from build123d import *

# Parameters (mm, degrees)
SKETCH_1_R          = 24
EXTRUDE_1_DEPTH     = 7
SKETCH_2_R          = 17
EXTRUDE_2_DEPTH     = 23
CUT_EXTRUDE_1_DEPTH = 23
CUT_EXTRUDE_3_REACH = 47.299
SKETCH_4_W          = 24
SKETCH_4_H          = 8.031532799
SKETCH_5_R          = 2
CUT_EXTRUDE_2_DEPTH = 42


with BuildPart() as part:
    # Эскиз1 → Вытянуть1 (new body)
    with BuildSketch(Plane(origin=(0, 0, 0), x_dir=(1, 0, 0), z_dir=(0, 1, 0))):
        with Locations(Location((0, 0, 0), (0, 0, 270))):
            Circle(SKETCH_1_R)
    extrude(amount=EXTRUDE_1_DEPTH)

    # Эскиз2 → Вытянуть2 (add)
    with BuildSketch(Plane(origin=(0, 7, 0), x_dir=(1, 0, 0), z_dir=(0, 1, 0))):
        with Locations(Location((0, 0, 0), (0, 0, 270))):
            Circle(SKETCH_2_R)
    extrude(amount=EXTRUDE_2_DEPTH)

    # Эскиз3 → Вырез-Вытянуть1 (cut, symmetric)
    with BuildSketch(Plane.XY):
        with BuildLine():
            Line((-7, 24.269678179), (7, 24.269678179))
            ThreePointArc((7, 24.269678179), (12, 19.269678179), (7, 14.269678179))
            Line((7, 14.269678179), (-7, 14.269678179))
            ThreePointArc((-7, 14.269678179), (-12, 19.269678179), (-7, 24.269678179))
        make_face()
    extrude(amount=CUT_EXTRUDE_1_DEPTH, both=True, mode=Mode.SUBTRACT)

    # Вытянуть3: up to this face of the body (flat: up to its plane)
    cut_extrude_3_end = Plane(part.part.faces().sort_by_distance((0, 7, -23.32117749))[0])
    # Эскиз4 → Вытянуть3 (cut, up to the picked face)
    with BuildSketch(Plane(origin=(0, 30, 0), x_dir=(-1, 0, 0), z_dir=(0, 1, 0)), mode=Mode.PRIVATE) as cut_extrude_3_sk1:
        with Locations((0, -16.0157664)):
            Rectangle(SKETCH_4_W, SKETCH_4_H)
    cut_extrude_3_tool1 = split(extrude(cut_extrude_3_sk1.sketch, amount=-CUT_EXTRUDE_3_REACH, mode=Mode.PRIVATE), bisect_by=cut_extrude_3_end, keep=Keep.BOTH, mode=Mode.PRIVATE)
    # Эскиз4 → Вытянуть3 (cut, up to the picked face)
    with BuildSketch(Plane(origin=(0, 30, 0), x_dir=(-1, 0, 0), z_dir=(0, 1, 0)), mode=Mode.PRIVATE) as cut_extrude_3_sk2:
        with Locations((0, 16.0157664)):
            Rectangle(SKETCH_4_W, SKETCH_4_H)
    cut_extrude_3_tool2 = split(extrude(cut_extrude_3_sk2.sketch, amount=-CUT_EXTRUDE_3_REACH, mode=Mode.PRIVATE), bisect_by=cut_extrude_3_end, keep=Keep.BOTH, mode=Mode.PRIVATE)
    add(cut_extrude_3_tool1.solids().sort_by(Axis((0, 30, -16.015766), (0, -1, 0)))[0], mode=Mode.SUBTRACT)
    add(cut_extrude_3_tool2.solids().sort_by(Axis((0, 30, 16.015766), (0, -1, 0)))[0], mode=Mode.SUBTRACT)

    # Эскиз5 → Вырез-Вытянуть2 (cut, through all)
    with BuildSketch(Plane(origin=(0, 7, 0), x_dir=(1, 0, 0), z_dir=(0, 1, 0))):
        with Locations(Location((0, 20, 0), (0, 0, 270))):
            Circle(SKETCH_5_R)
        with Locations(Location((17.320508076, 10, 0), (0, 0, 270))):
            Circle(SKETCH_5_R)
        with Locations(Location((17.320508076, -10, 0), (0, 0, 270))):
            Circle(SKETCH_5_R)
        with Locations(Location((0, -20, 0), (0, 0, 270))):
            Circle(SKETCH_5_R)
        with Locations(Location((-17.320508076, -10, 0), (0, 0, 270))):
            Circle(SKETCH_5_R)
        with Locations(Location((-17.320508076, 10, 0), (0, 0, 270))):
            Circle(SKETCH_5_R)
    extrude(amount=-CUT_EXTRUDE_2_DEPTH, mode=Mode.SUBTRACT)


solid = part.part
Can you work these out from the model? Positions are in its coordinate system, mm. A direction names the side the tool comes from. Round coordinates to 2 decimals unless told otherwise and drop trailing zeros. Loops run counter-clockwise (first coordinate to the right, second up) from the corner with the lowest first, then second, coordinate; pieces in that order, holes last. Notation, with made-up numbers: (-6, -32.75) - (12, -32.75) arc R23 ccw to (12, -9.75) - close; hole circle Ø4 at (89, 4). An arc over 180 degrees is marked (long way). Answer in a Markdown table with one row per item. Add a question column.
Q1. I want a section at C-C on x = 18.5. List the corners of the cut face in (y, z) for me, and give its area (3 significant figures).
Q2. For pin 1 Ø2 at (y, z) = (3, 3) entering from +X; pin 2 Ø5 at (x, z) = (0, 20) entering from +Y; pin 3 Ø3 at (x, y) = (1, 25) entering from +Z, each with a flat end and sliding along its axis, tell me the tip position at first contact or that it passes through.
Q3. I need wall thicknesses on L1, parallel to Y at x = 6.5, z = -2.5; L2, parallel to X at y = 6.5, z = 10.5; L3, parallel to Y at x = -6, z = 21.5. Which ranges of each line are inside material? Lowest first, please.
Q4. I want a section at D-D on z = 19. List the corners of the cut face in (x, y) for me, and give its area (3 significant figures).
Q5. Which directions (+Z, -Z, +X, -X, +Y, -Y) give clear straight access to the entire face, cutting with the end or side of a thin tool? Please do faces 4 (the flat face through (0, 24.27, 0)), 5 (the cylindrical face through (-17, 18, 0)).
Q6. We'd pull the mould along Y, two halves only. Please class faces 1 (the cylindrical face through (12, 19.4, 0.2)), 2 (the flat face through (0, 0, 0)), 3 (the cylindrical face through (17, 18, 0)): pulls with the +Y half, pulls with the -Y half, needs draft (parallel to the pull), parting line crosses it, or undercut.
Q7. I want a section at B-B on x = 0. List the corners of the cut face in (y, z) for me, and give its area (3 significant figures).
Q8. I want a section at A-A on z = -10. List the corners of the cut face in (x, y) for me, and give its area (3 significant figures).
A:
| question | item | result |
|---|---|---|
| 1 | outline | (0, -15.29) - (7, -15.29) - (7, -11.62) - (0, -11.62) - close; (0, -8.38) - (7, -8.38) - (7, 8.38) - (0, 8.38) - close; (0, 11.62) - (7, 11.62) - (7, 15.29) - (0, 15.29) - close |
| 1 | area | 169 mm^2 |
| 2 | pin 1 | x = 23.92 |
| 2 | pin 2 | y = 7 |
| 2 | pin 3 | z = 12 |
| 3 | L1 | 0 to 14.27, 24.27 to 30 |
| 3 | L2 | -21.58 to -19.26, -15.38 to 15.38, 19.26 to 21.58 |
| 3 | L3 | 0 to 7 |
| 4 | outline | (-14.66, 0) - (-1.73, 0) - (-1.73, 7) - (-14.66, 7) - close; (1.73, 0) - (14.66, 0) - (14.66, 7) - (1.73, 7) - close |
| 4 | area | 181 mm^2 |
| 5 | face 4 | +Z, -Z |
| 5 | face 5 | -X, +Y |
| 6 | face 1 | undercut |
| 6 | face 2 | pulls with the -Y half |
| 6 | face 3 | needs draft |
| 7 | outline | (0, -24) - (7, -24) - (7, -22) - (0, -22) - close; (0, -18) - (7, -18) - (7, -12) - (14.27, -12) - (14.27, 12) - (7, 12) - (7, 18) - (0, 18) - close; (0, 22) - (7, 22) - (7, 24) - (0, 24) - close; (24.27, -12) - (30, -12) - (30, 12) - (24.27, 12) - close |
| 7 | area | 592 mm^2 |
| 8 | outline | (-21.82, 0) - (-19.32, 0) - (-19.32, 7) - (-21.82, 7) - close; (-15.32, 0) - (15.32, 0) - (15.32, 7) - (13.75, 7) - (13.75, 30) - (-13.75, 30) - (-13.75, 7) - (-15.32, 7) - close; (19.32, 0) - (21.82, 0) - (21.82, 7) - (19.32, 7) - close; hole (-7, 14.27) - (7, 14.27) arc R5 ccw to (7, 24.27) - (-7, 24.27) arc R5 ccw to start |
| 8 | area | 663 mm^2 |
